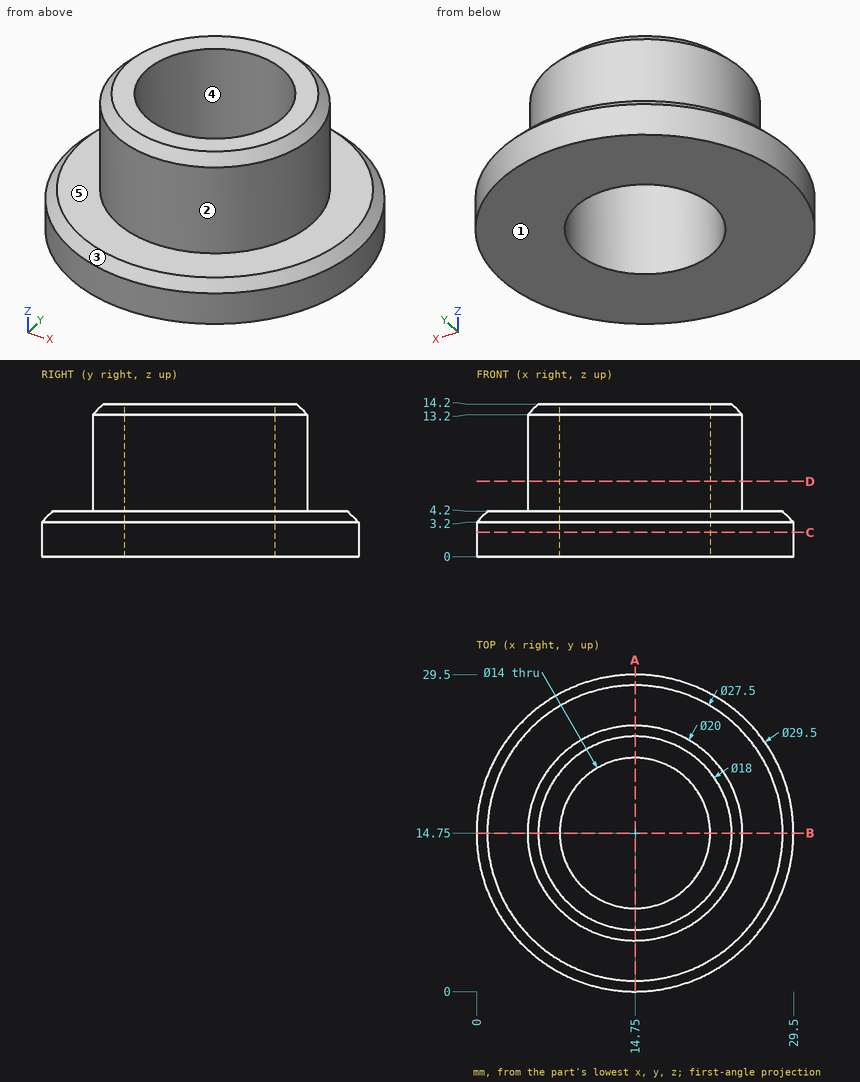
Part print with two shaded views. Sizes in mm from the minimum x, y, z corner. A direction names the side the tool comes from. Round coordinates to 2 decimals unless told otherwise and drop trailing zeros. Order: outer loops, then holes, each group sorted by start corner. A loop starts at its lowest first (then second) coordinate and runs counter-clockwise, first axis right, second up.
(1) Band-saw the part on A-A (x = 14.75). List the corners of the cut face in (y, z).
(2) Band-saw the part on C-C (z = 2.25). List the corners of the cut face in (x, y), then the cut area to 3 significant figures.
(3) 3-axis set-ups, long thin cutter, end or side, ignore diameter. For the marked faces 1 and 2: which of +Z, -Z, +X, -X, +Y, -Y reach the whole face in a straight line?
(4) Drill centre lines: line 1 (Y direction, x = 14.75, z = 6.5); line 2 (Z direction, x = 13.25, y = 3.75); line 3 (Y direction, x = 9.75, z = 4.75). Where is each one in solid material? Low to high.
(5) Pull direction X, two halves, no side cores. Call the marked faces 3, 4 and 5: released by +X, released by -X, zero draft, split by the parting line, or undercut.
(6) Pin check, flat tips, straight feed: pin 1 (2 mm diameter, centred on x = 24.5, z = 5, fed in from +Y); pin 2 (1 mm diameter, centred on x = 9, z = 11, fed in from -Y); pin 3 (1.5 mm diameter, centred on x = 7, z = 2, fed in from +Y). Stop position of each tip, or through.
(7) Band-saw the part on D-D (z = 7). List the corners of the cut face in (x, y), then the cut area to 3 significant figures.
Verdict:
1. outline: (0, 0) - (7.75, 0) - (7.75, 14.2) - (5.75, 14.2) - (4.75, 13.2) - (4.75, 4.2) - (1, 4.2) - (0, 3.2) - close; (21.75, 0) - (29.5, 0) - (29.5, 3.2) - (28.5, 4.2) - (24.75, 4.2) - (24.75, 13.2) - (23.75, 14.2) - (21.75, 14.2) - close
2. outline: circle Ø29.5 at (14.75, 14.75); hole circle Ø14 at (14.75, 14.75)
2. area: 530 mm2
3. face 1: -Z, +X, -X, +Y, -Y
3. face 2: +Z
4. line 1: y = 4.75 to 7.75, 21.75 to 24.75
4. line 2: z = 0 to 4.2
4. line 3: y = 6.09 to 9.85, 19.65 to 23.41
5. face 3: split by the parting line
5. face 4: undercut
5. face 5: zero draft
6. pin 1: stops at y = 25.02
6. pin 2: stops at y = 6.24
6. pin 3: stops at y = 27.73
7. outline: circle Ø20 at (14.75, 14.75); hole circle Ø14 at (14.75, 14.75)
7. area: 160 mm2
